The drawing under review shows one solid part. Ordinate dimensions are in mm from its lowest x, y, z. A direction names the side the tool comes from. Coordinates: 2 decimals unless noted, no trailing zeros. Loops run counter-clockwise (first coordinate to the right, second up) from the corner with the lowest first, then second, coordinate; pieces in that order, holes last. Notation, with made-up numbers: M -8.75,87.25 L 31.25,87.25 A28 ccw 31.25,107.25 Z; hole C 5,36.5 d4. An arc over 180 degrees is marked long. Return JSON: item names as keys, results as strings.
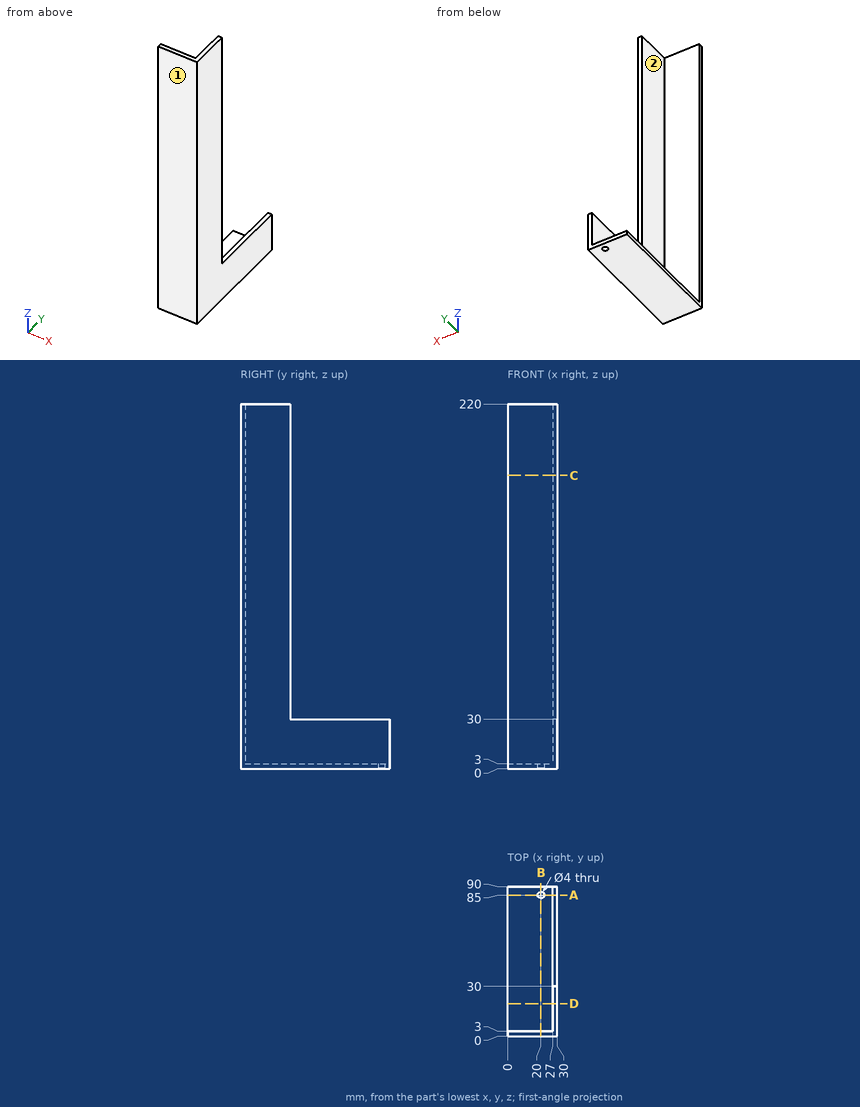
1. Add section D-D on y = 19.5. Give the boundary of the cut face in (x, z), plus the area to 3 significant figures.
Check values:
{"outline": "M 0,0 L 30,0 L 30,220 L 27,220 L 27,3 L 0,3 Z", "area": "741 mm²"}
2. Add section C-C on z = 177. Give the boundary of the cut face in (x, y).
Check values:
{"outline": "M 0,0 L 30,0 L 30,30 L 27,30 L 27,3 L 0,3 Z"}
3. To check wall thickness, follow line 1 (Y direction, x = 20, z = 1.5); line 2 (Z direction, x = 7.5, y = 16). State the ranges of each line that lie inside material, in increasing order.
Check values:
{"line 1": "0 to 83, 87 to 90", "line 2": "0 to 3"}
4. Machinability: for the marked faces 1 and 2, which of the approach directions +Z, -Z, +X, -X, +Y, -Y give a long, thin tool a straight path to every point of the face, cutting with its end or side? Answer none if there is none.
Check values:
{"face 1": "+Z, -Z, +X, -X, -Y", "face 2": "+Z, -X, +Y"}
5. Add section A-A on y = 85. Give the boundary of the cut face in (x, z), plus the area to 3 significant figures.
Check values:
{"outline": "M 0,0 L 18,0 L 18,3 L 0,3 Z; M 22,0 L 30,0 L 30,30 L 27,30 L 27,3 L 22,3 Z", "area": "159 mm²"}
6. Add section B-B on x = 20. Give the boundary of the cut face in (y, z), plus the area to 3 significant figures.
Check values:
{"outline": "M 0,0 L 83,0 L 83,3 L 3,3 L 3,220 L 0,220 Z; M 87,0 L 90,0 L 90,3 L 87,3 Z", "area": "909 mm²"}
7. Insertion check: pin 1 Ø10 at (x, y) = (17.5, 53.5) entering from +Z; pin 2 Ø1 at (x, z) = (22, 134) entering from +Y; pin 3 Ø3.5 at (x, z) = (28.5, 83.5) entering from +Y. Each pin has a flat end and moves straight along its axis. Give the tip position at first contact, or say it passes through.
Check values:
{"pin 1": "z = 3", "pin 2": "y = 3", "pin 3": "y = 30"}
